Check sheet for the modelled part. Datum: model origin and axes. Units: mm. A direction names the side the tool comes from. Give positions to 0.01 mm unless a question says otherwise; leave off trailing zeros. Loops run counter-clockwise (first coordinate to the right, second up) from the corner with the lowest first, then second, coordinate; pieces in that order, holes last. Notation, with made-up numbers: (22.5, 33.25) -> (59.5, 33.25) arc R12 ccw to (59.5, 50.25) -> close; hole circle Ø7 at (19.5, 1). An arc over 180 degrees is marked (long way). Write each question's results on one line, items separated by ' | '. Start each with the question number.
1. Material ranges on L1, parallel to X at y = -2.5, z = -1.5; L2, parallel to Y at x = 0, z = 2.6; L3, parallel to Y at x = 1.5, z = 2.75, recorded low to high. Write a range as from..to.
2. Cross-section at C-C on x = 0. Record the boundary of the cut face in (y, z).
3. Cross-section at D-D on z = -2.25. Record the boundary of the cut face in (x, y).
4. Mould release check, pull along X, two halves, no side actions. Record for faces 1 (the face through (-8.699, -6.07, 3.215)), 2 (the face through (6.2, -6, -1)), 3 (the face through (-1, 0, 2)): +X half, -X half, draft (parallel to the pull), parting line (faces both ways), or undercut.
5. Gauge pin test, flat end, axial feed: pin 1 Ø4.5 at (x, y) = (0, -6) entering from -Z. Record the tip position at first contact, or that the pin passes through.
6. Cross-section at A-A on z = 1.75. Record the boundary of the cut face in (x, y).
7. Tool access check on faces 4 (the face through (6.501, -0.285, -1.035)), 5 (the face through (-7.208, -0.285, -3.199)), 6 (the face through (-6.301, -11.715, -0.965)). Record the directions out of +Z, -Z, +X, -X, +Y, -Y that give a thin tool (end or side, any length) a straight path to the whole face; none if there is none.
8. Cross-section at B-B on y = -6. Record the boundary of the cut face in (x, z), and give its area (3 significant figures).
from build123d import *

# Parameters (mm, degrees)
F1_DEPTH = 12
F2_R     = 1.7
F3_DEPTH = 7.001
F2_R_2   = 2.9
F4_DEPTH = 2
F5_R     = 1


with BuildPart() as f1:
    # F0 (on Front) → F1 (new body)
    with BuildSketch(Plane.XZ):
        Polygon((9, -3.5), (9, 3.5), (-9, 3.5), (-9, -3.5), (-6, -3.5), (-6, 0.5), (6.2, 0.5), (6.2, -3.5), align=None)
    extrude(amount=F1_DEPTH)

    # F2 (on face) → F3 (cut, through all)
    with BuildSketch(Plane.XY.offset(3.5)):
        with Locations((0, -6)):
            Circle(F2_R)
    extrude(amount=-F3_DEPTH, mode=Mode.SUBTRACT)

    # F2 (on face) → F4 (cut)
    with BuildSketch(Plane.XY.offset(3.5)):
        with Locations((0, -6)):
            Circle(F2_R_2)
        with Locations((0, -6)):
            Circle(F2_R, mode=Mode.SUBTRACT)
    extrude(amount=-F4_DEPTH, mode=Mode.SUBTRACT)

    # F5
    f5_edges = [f1.edges().sort_by_distance(p)[0] for p in [
        (9, -12, 0),
        (0, -12, 3.5),
        (-9, -12, 0),
        (-7.5, -12, -3.5),
        (-6, -12, -1.5),
        (0.1, -12, 0.5),
        (6.2, -12, -1.5),
        (7.6, -12, -3.5),
        (9, 0, 0),
        (0, 0, 3.5),
        (-9, 0, 0),
        (-7.5, 0, -3.5),
        (-6, 0, -1.5),
        (0.1, 0, 0.5),
        (6.2, 0, -1.5),
        (7.6, 0, -3.5),
        (9, -6, -3.5),
        (-9, -6, -3.5),
        (-9, -6, 3.5),
        (9, -6, 3.5),
    ]]
    fillet(f5_edges, radius=F5_R)


solid = f1.part
Geometry says:
1) L1: -9..-6, 6.2..9 | L2: -11.99..-8.9, -3.1..-0.01 | L3: -11.97..-8.48, -3.52..-0.03
2) outline: (-12, 1.5) arc R1 ccw to (-11, 0.5) -> (-7.7, 0.5) -> (-7.7, 1.5) -> (-8.9, 1.5) -> (-8.9, 3.5) -> (-11, 3.5) arc R1 ccw to (-12, 2.5) -> close; (-4.3, 0.5) -> (-1, 0.5) arc R1 ccw to (0, 1.5) -> (0, 2.5) arc R1 ccw to (-1, 3.5) -> (-3.1, 3.5) -> (-3.1, 1.5) -> (-4.3, 1.5) -> close
3) outline: (-9, -11) arc R1 ccw to (-8, -12) -> (-7, -12) arc R1 ccw to (-6, -11) -> (-6, -1) arc R1 ccw to (-7, 0) -> (-8, 0) arc R1 ccw to (-9, -1) -> close; (6.2, -11) arc R1 ccw to (7.2, -12) -> (8, -12) arc R1 ccw to (9, -11) -> (9, -1) arc R1 ccw to (8, 0) -> (7.2, 0) arc R1 ccw to (6.2, -1) -> close
4) face 1: -X half | face 2: undercut | face 3: draft
5) pin 1: z = 0.5
6) outline: (-9, -11) arc R1 ccw to (-8, -12) -> (8, -12) arc R1 ccw to (9, -11) -> (9, -1) arc R1 ccw to (8, 0) -> (-8, 0) arc R1 ccw to (-9, -1) -> close; hole circle Ø5.8 at (0, -6)
7) face 4: -Z, +Y | face 5: -Z, +X, -X, +Y | face 6: -Z, -Y
8) outline: (-9, -2.5) arc R1 ccw to (-8, -3.5) -> (-6, -3.5) -> (-6, 0.5) -> (-1.7, 0.5) -> (-1.7, 1.5) -> (-2.9, 1.5) -> (-2.9, 3.5) -> (-8, 3.5) arc R1 ccw to (-9, 2.5) -> close; (1.7, 0.5) -> (6.2, 0.5) -> (6.2, -3.5) -> (8, -3.5) arc R1 ccw to (9, -2.5) -> (9, 2.5) arc R1 ccw to (8, 3.5) -> (2.9, 3.5) -> (2.9, 1.5) -> (1.7, 1.5) -> close | area: 61.3 mm^2
